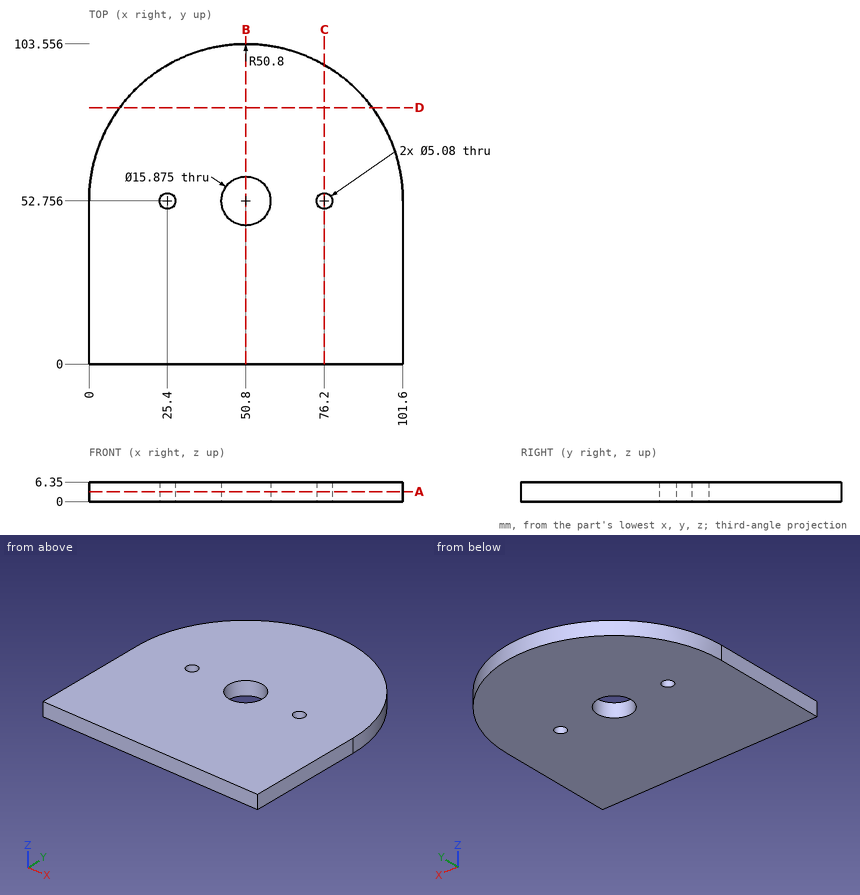
Input: dimensioned drawing with shaded views. Units: mm. Origin: part minimum x, y, z. Round coordinates to 2 decimals unless told otherwise and drop trailing zeros. Loops run counter-clockwise (first coordinate to the right, second up) from the corner with the lowest first, then second, coordinate; pieces in that order, holes last. Notation, with made-up numbers: (-36, 74.25) -> (3, 74.25) arc R14 ccw to (3, 80.25) -> close; hole circle Ø3 at (25.25, 87.5). An arc over 180 degrees is marked (long way). Answer as a JSON object with one key per item and string values. Group by question number.
1) Section query A-A on z = 3.25. Output: boundary loops of the cut face in (x, y) (1 decimal).
2) Section query D-D on y = 83. Output: boundary loops of the cut face in (x, z), plus the area to 3 significant figures.
3) Pin query (flat end, axial travel): pin 1 (4 mm diameter, centred on x = 10, y = 79.5, fed in from -Z); pin 2 (3 mm diameter, centred on y = 73, z = 5, fed in from +X) (1 decimal). Return the tip coordinate at first contact, or that it passes through.
4) Section query C-C on x = 76.2. Output: boundary loops of the cut face in (y, z).
5) Section query B-B on x = 50.8. Output: boundary loops of the cut face in (y, z).
6) Ray query, L1, parallel to X at y = 52.5, z = 4; L2, parallel to Y at x = 50.8, z = 3.25; L3, parallel to X at y = 52, z = 2.5 (1 decimal). Return the intervals inside material, ascending.
Reply:
{
 "1": {"outline": "(0, 0) -> (101.6, 0) -> (101.6, 52.8) arc R50.8 ccw to (0, 52.8) -> close; hole circle Ø5.1 at (25.4, 52.8); hole circle Ø15.9 at (50.8, 52.8); hole circle Ø5.1 at (76.2, 52.8)"},
 "2": {"outline": "(9.98, 0) -> (91.62, 0) -> (91.62, 6.35) -> (9.98, 6.35) -> close", "area": "518 mm2"},
 "3": {"pin 1": "stops at z = 0", "pin 2": "stops at x = 98"},
 "4": {"outline": "(0, 0) -> (50.22, 0) -> (50.22, 6.35) -> (0, 6.35) -> close; (55.3, 0) -> (96.75, 0) -> (96.75, 6.35) -> (55.3, 6.35) -> close"},
 "5": {"outline": "(0, 0) -> (44.82, 0) -> (44.82, 6.35) -> (0, 6.35) -> close; (60.69, 0) -> (103.56, 0) -> (103.56, 6.35) -> (60.69, 6.35) -> close"},
 "6": {"L1": "x = 0 to 22.87, 27.93 to 42.87, 58.73 to 73.67, 78.73 to 101.6", "L2": "y = 0 to 44.82, 60.69 to 103.56", "L3": "x = 0 to 23, 27.8 to 42.9, 58.7 to 73.8, 78.6 to 101.6"}
}
